Model file for the job. Use its own axes, mm. A direction names the side the tool comes from. Give positions to 0.01 mm unless a question says otherwise; leave off trailing zeros. Write each loop counter-clockwise with the first axis right and the second up, starting at its lowest first coordinate (ties: lowest second). Pieces come first, ordered by that corner, then holes.
Autodesk Inventor part; units mm, degrees
ref_plane "YZ Plane" through (0, 0, 0) normal (1, 0, 0) x (0, 1, 0)
ref_plane "XZ Plane" through (0, 0, 0) normal (0, 1, 0) x (-1, 0, 0)
ref_plane "XY Plane" through (0, 0, 0) normal (0, 0, 1) x (1, 0, 0)
sketch "Sketch1" plane through (0, 0, 0) normal (0, 0, 1) x (1, 0, 0)
  line L0 (-35, 0) -> (-35, 12)
  line L1 (-35, 12) -> (24, 12)
  line L2 (24, 12) -> (24, 0)
  line L3 (24, 0) -> (10, 0)
  line L4 (10, 0) -> (10, 3.1)
  line L5 (10, 3.1) -> (-14, 3.1)
  line L6 (-14, 3.1) -> (-14, 0)
  line L7 (-14, 0) -> (-35, 0)
  line L8 (0, 0) -> (0, 12) construction
  line L9 (-14, 0) -> (0, 0) construction
  dimension "d0" = 3.1
  dimension "d1" = 24
  dimension "d3" = 12
  dimension "d7" = 10
  dimension "d8" = 24
  dimension "d9" = 35
extrude "Extrusion1" add sketch "Sketch1" along normal blind 3
fillet "Fillet1" radius 2 2 edges at (-35, 12, 1.5) (24, 12, 1.5)
properties part number "shovel_support"
1. Pin check, flat tip, straight feed: P1, Ø1.5, axis at x = -1.5, z = 2, coming from the -Y side. Stop position of the tip, or through.
Calculated:
P1: stops at y = 3.1
2. Pull direction X, two halves, no side cores. Call faces 3 (the flat face through (17, 0, 1)), 4 (the flat face through (24, 5, 1)), 5 (the flat face through (-35, 5, 1)), 6 (the flat face through (-14, 2, 1)): +X half, -X half, draft (parallel to the pull), parting line (faces both ways), or undercut.
Calculated:
face 3: draft
face 4: +X half
face 5: -X half
face 6: undercut
3. Slice it at B-B, the plane x = -5.5. Write the cut outline in (y, z).
Calculated:
outline: (3.1, 0) - (12, 0) - (12, 3) - (3.1, 3) - close
4. Slice it at A-A, the plane z = 0.75. Write the cut outline in (x, y), and give its area (3 significant figures).
Calculated:
outline: (-35, 0) - (-14, 0) - (-14, 3.1) - (10, 3.1) - (10, 0) - (24, 0) - (24, 10) arc R2 ccw to (22, 12) - (-33, 12) arc R2 ccw to (-35, 10) - close
area: 632 mm2
5. Probe probe 1 along X at (y, z) = (2, 0.4); probe 2 along Y at (x, z) = (-2, 1.6); probe 3 along X at (y, z) = (10.5, 2.3). List the from-to ranges inside material, lowest first.
Calculated:
probe 1: x = -35 to -14, 10 to 24
probe 2: y = 3.1 to 12
probe 3: x = -34.94 to 23.94
6. Which spindle directions (+Z, -Z, +X, -X, +Y, -Y) get a long thin tool onto all of the face, cutting with end or side? Do faces 1 (the flat face through (-2, 3.1, 1)), 2 (the cylindrical face through (23.43, 11.4, 1.52)). Say none if no direction does.
Calculated:
face 1: +Z, -Z, -Y
face 2: +Z, -Z, +X, +Y
